Can you work these out from the model? Positions are in its coordinate system, mm. Give positions to 0.01 mm unless a question says otherwise; leave off trailing zeros. Order: outer loops, then holes, each group sorted by start corner. A loop starts at its lowest first (then second) coordinate and runs counter-clockwise, first axis right, second up. Notation, with made-up numbers: (51, 39.25) -> (65, 39.25) arc R16 cw to (65, 67.25) -> close; hole circle Ø7 at (47, -29.5). An arc over 180 degrees is marked (long way). Answer as CSV lines item,"result".
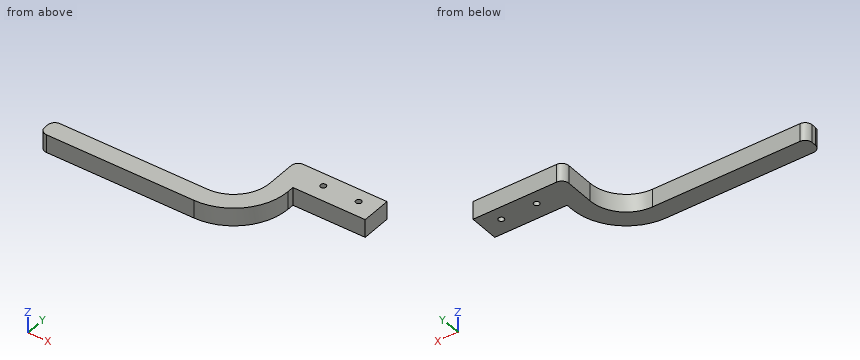
```python
from build123d import *

# Parameters (mm, degrees)
BOSS_EXTRUDE1_DEPTH = 12.7
FILLET1_R           = 5
SKETCH2_R           = 2
CUT_EXTRUDE1_DEPTH  = 13.7


with BuildPart() as part:
    # Sketch1 → Boss-Extrude1 (new body)
    with BuildSketch(Plane.XY):
        with BuildLine():
            Line((0, 0), (-64, 0))
            Line((-64, 0), (-64, -25.552169744))
            ThreePointArc((-64, -25.552169744), (-71.453496915, -43.546503085), (-89.447830256, -51))
            Line((-89.447830256, -51), (-198.447830256, -51))
            Line((-198.447830256, -51), (-198.447830256, -63.95586098))
            Line((-198.447830256, -63.95586098), (-89.447830256, -63.95586098))
            ThreePointArc((-89.447830256, -63.95586098), (-62.29231976, -52.70768024), (-51.04413902, -25.552169744))
            Line((-51.04413902, -25.552169744), (-51.04413902, -21))
            Line((-51.04413902, -21), (0, -21))
            Line((0, -21), (0, 0))
        make_face()
    extrude(amount=BOSS_EXTRUDE1_DEPTH)

    # Fillet1
    fillet1_edges = [part.edges().sort_by_distance(p)[0] for p in [
        (-198.447830256, -63.95586098, 6.35),
        (-198.447830256, -51, 6.35),
        (-64, 0, 6.35),
    ]]
    fillet(fillet1_edges, radius=FILLET1_R)

    # Sketch2 → Cut-Extrude1 (cut, through all)
    with BuildSketch(Plane.XY.offset(12.7)):
        with Locations((-13, -9.531609903)):
            Circle(SKETCH2_R)
        with Locations((-38, -9.531609903)):
            Circle(SKETCH2_R)
    extrude(amount=-CUT_EXTRUDE1_DEPTH, mode=Mode.SUBTRACT)


solid = part.part
```
Item 1: Please list where these lines run through material, in increasing order: line 1 along Y through (x, z) = (-38, 9.25); line 2 along X through (y, z) = (-10, 8.75); line 3 along Y through (x, z) = (-188.5, 1.5).
Numbers:
line 1,"y = -21 to -11.53, -7.53 to 0"
line 2,"x = -64 to -39.94, -36.06 to -14.94, -11.06 to 0"
line 3,"y = -63.96 to -51"
Item 2: Imagine slicing it at B-B, the plane z = 4. Please give me the cut outline in (x, y).
Numbers:
outline,"(-198.45, -58.96) arc R5 ccw to (-193.45, -63.96) -> (-89.45, -63.96) arc R38.4 ccw to (-51.04, -25.55) -> (-51.04, -21) -> (0, -21) -> (0, 0) -> (-59, 0) arc R5 ccw to (-64, -5) -> (-64, -25.55) arc R25.45 cw to (-89.45, -51) -> (-193.45, -51) arc R5 ccw to (-198.45, -56) -> close; hole circle Ø4 at (-38, -9.53); hole circle Ø4 at (-13, -9.53)"
Item 3: Imagine slicing it at A-A, the plane x = -13. Please give me the cut outline in (y, z), then the cut area to 3 significant figures.
Numbers:
outline,"(-21, 0) -> (-11.53, 0) -> (-11.53, 12.7) -> (-21, 12.7) -> close; (-7.53, 0) -> (0, 0) -> (0, 12.7) -> (-7.53, 12.7) -> close"
area,"216 mm²"
Item 4: Imagine slicing it at C-C, the plane x = -42. Please give me the cut outline in (y, z), then the cut area to 3 significant figures.
Numbers:
outline,"(-21, 0) -> (0, 0) -> (0, 12.7) -> (-21, 12.7) -> close"
area,"267 mm²"
Item 5: For pin 1 (4 mm diameter, centred on x = -58.5, z = 8, fed in from -Y); pin 2 (3 mm diameter, centred on y = -25, z = 4, fed in from +X); pin 3 (4.5 mm diameter, centred on x = -13, y = -9.53, fed in from +Z); pin 4 (1.5 mm diameter, centred on y = -27.5, z = 4, fed in from -X), each with a flat end and sliding along its axis, tell me the tip position at first contact or that it passes through.
Numbers:
pin 1,"stops at y = -50.79"
pin 2,"stops at x = -51.04"
pin 3,"stops at z = 12.7"
pin 4,"stops at x = -64.14"
Item 6: Imagine slicing it at D-D, the plane y = -47.5. Please give me the cut outline in (x, z), then the cut area to 3 significant figures.
Numbers:
outline,"(-76.57, 0) -> (-57.93, 0) -> (-57.93, 12.7) -> (-76.57, 12.7) -> close"
area,"237 mm²"
